Autodesk Inventor part; units mm, degrees
ref_plane "YZ Plane" through (0, 0, 0) normal (1, 0, 0) x (0, 1, 0)
ref_plane "XZ Plane" through (0, 0, 0) normal (0, 1, 0) x (-1, 0, 0)
ref_plane "XY Plane" through (0, 0, 0) normal (0, 0, 1) x (1, 0, 0)
sketch "Sketch1" plane through (0, 0, 0) normal (0, 1, 0) x (-1, 0, 0)
  line L0 (0, 0) -> (-132.537, 0) construction
  line L1 (0, 4) -> (-132.537, 4)
  line L2 (-132.537, -4) -> (0, -4)
  arc A0 (0, -4) -> (0, 4) centre (0, 0) ccw
  arc A1 (-132.537, 4) -> (-132.537, -4) centre (-132.537, 0) ccw
  circle A2 centre (0, 0) radius 2.1
  circle A3 centre (-16.286, 0) radius 2.1
  circle A4 centre (-132.537, 0) radius 2.1
  circle A5 centre (-107.252, 0) radius 2.1
  point P0 (-66.2685, 0)
  point P1 (-52.7225, 0)
  dimension "d0" = 132.537
  dimension "d1" = 8
  dimension "d2" = 4.2
  dimension "d8" = 4.2
  dimension "d9" = 16.286
  dimension "d10" = 4.2
  dimension "d28" = 4.2
  dimension "d29" = 107.252
extrude "Extrusion1" add sketch "Sketch1" along normal blind 5
sketch "Sketch4" plane through (0, 5, 0) normal (0, 1, 0) x (1, 0, 0)
  arc A0 (132.537, -4) -> (132.537, 4) centre (132.537, 0) ccw
  line L0 (132.537, 4) -> (0, 4)
  arc A1 (0, 4) -> (0, -4) centre (0, 0) ccw
  line L1 (0, -4) -> (132.537, -4)
  circle A2 centre (16.286, 0) radius 2.1
  circle A3 centre (107.252, 0) radius 2.1
  circle A4 centre (132.537, 0) radius 2.1
  circle A5 centre (0, 0) radius 2.1
  circle A6 centre (16.286, 0) radius 4
  dimension "d30" = 8
extrude "Extrusion7" add sketch "Sketch4" along normal blind 5 contours A6
Design review of the part built by this model. Coordinates are the model's own, in mm. Give positions to 0.01 mm unless a question says otherwise; leave off trailing zeros. Order: outer loops, then holes, each group sorted by start corner. A loop starts at its lowest first (then second) coordinate and runs counter-clockwise, first axis right, second up. Notation, with made-up numbers: (-13, 67.25) - (24, 67.25) arc R16 ccw to (24, 95.25) - close; hole circle Ø8 at (22, 51). An arc over 180 degrees is marked (long way). Use a Markdown table: item, result. Add a question column.
(1) Clearance check with flat-ended pins moving along their axes: P1, Ø4, axis at x = 24, z = 1.5, coming from the +Y side; P2, Ø4, axis at x = 16.286, z = 0, coming from the -Y side. State where each tip first meets the part, or that it passes through.
(2) Add section A-A on y = 3.25. Give the boundary of the cut face in (x, z).
(3) Mouldability with a two-part tool opening along X and no side actions: class faces 1 (the face through (136.536, 2.465, -0.088)), 2 (the face through (67, 2, -4)), 3 (the face through (18.13, 7.46, -3.55)), 4 (the face through (-2.003, 2.465, -0.631)) as +X half, -X half, draft (parallel to the pull), parting line (faces both ways), or undercut.
(4) Add section B-B on x = 97.5. Give the boundary of the cut face in (y, z), then the cut area to 3 significant figures.
(5) Wall thickness on probe 1 along X at (y, z) = (7.25, 0); probe 2 along Y at (x, z) = (34.5, -3.5); probe 3 along X at (y, z) = (4.5, 1): over which ranges is each line inside the solid? List them lowest first. Write a range as [from, to].
Report:
| question | item | result |
|---|---|---|
| 1 | P1 | stops at y = 5 |
| 1 | P2 | passes through |
| 2 | outline | (0, -4) - (132.54, -4) arc R4 ccw to (132.54, 4) - (0, 4) arc R4 ccw to start; hole circle Ø4.2 at (0, 0); hole circle Ø4.2 at (16.29, 0); hole circle Ø4.2 at (107.25, 0); hole circle Ø4.2 at (132.54, 0) |
| 3 | face 1 | +X half |
| 3 | face 2 | draft |
| 3 | face 3 | parting line |
| 3 | face 4 | undercut |
| 4 | outline | (0, -4) - (5, -4) - (5, 4) - (0, 4) - close |
| 4 | area | 40.0 mm² |
| 5 | probe 1 | x = [12.29, 14.19], [18.39, 20.29] |
| 5 | probe 2 | y = [0, 5] |
| 5 | probe 3 | x = [-3.87, -1.85], [1.85, 14.44], [18.13, 105.41], [109.1, 130.69], [134.38, 136.41] |
